Design review of the part built by this model. Coordinates are the model's own, in mm. A direction names the side the tool comes from. Give positions to 0.01 mm unless a question says otherwise; leave off trailing zeros. Order: outer loops, then holes, each group sorted by start corner. A loop starts at its lowest first (then second) coordinate and runs counter-clockwise, first axis right, second up. Notation, with made-up numbers: (64.25, 42.5) -> (77.25, 42.5) arc R16 ccw to (77.25, 51.5) -> close; hole circle Ø10 at (25, 60.25). An arc over 180 degrees is marked (long way). One line per item, written item: value. Start each with the question number.
1) The part is to be moulded in two halves that separate along Y. For faces 1 (the face through (2.958, 6.293, -6.36)), 2 (the face through (2.958, 3.735, 8.095)), 3 (the face through (2.958, -8.064, -3.8)), say which applies: released by +Y, released by -Y, zero draft, split by the parting line, or undercut.
2) Wall thickness on line 1 along Y through (x, z) = (2.1, 0); line 2 along Y through (x, z) = (0.35, 9.25); line 3 along Z through (x, y) = (2.05, 8.25): over which ranges is each line inside the solid? List them lowest first. Write a range as from..to.
3) Consider section D-D (y = 4). State the section outline as (x, z) points, plus the area to 3 significant figures.
4) Tool access review of faces 4 (the face through (2.96, -7.75, 0.01)), 5 (the face through (2.958, -3.881, -6.707)), 6 (the face through (2.958, 8.878, 0.813)), 7 (the face through (2.96, -2.34, 8.6)), 8 (the face through (6, 2.1, 2.4)): name each direction out of +Z, -Z, +X, -X, +Y, -Y from which nothing blocks a thin tool from reaching the whole face with its end or side.
5) Consider section B-B (y = 0). State the section outline as (x, z) points.
6) Consider section C-C (z = -3.75). State the section outline as (x, y) points.
7) Consider section A-A (z = 0). State the section outline as (x, y) points, plus the area to 3 significant figures.
from build123d import *

# Parameters (mm, degrees)
BASPROSKE_W        = 6
BASPROSKE_H        = 10
TOOTHCUT_DEPTH     = 16.362291496
TEETHCUTS_COUNT    = 18
TEETHCUTS_ANGLE    = 340
CUT_EXTRUDE1_DEPTH = 16.289512146


with BuildPart() as part:
    # BasProSke → Base-Revolve (revolve)
    with BuildSketch(Plane(origin=(0, 0, 0), x_dir=(1, 0, 0), z_dir=(0, 1, 0)), mode=Mode.PRIVATE) as base_revolve_sk:
        with Locations((3, 5)):
            Rectangle(BASPROSKE_W, BASPROSKE_H)
    revolve(base_revolve_sk.sketch.rotate(Axis((-10, 0, 0), (1, 0, 0)), 180), axis=Axis((-10, 0, 0), (1, 0, 0)))

    # TooCutSke → ToothCut (cut, through all)
    with BuildSketch(Plane(origin=(0, 0, 0), x_dir=(0, 0, -1), z_dir=(1, 0, 0))):
        with BuildLine():
            ThreePointArc((0.510641536, 7.732156635), (0, 7.749), (-0.510641536, 7.732156635))
            ThreePointArc((-0.510641536, 7.732156635), (-0.82619259, 8.907320741), (-1.515208602, 9.910236529))
            ThreePointArc((-1.515208602, 9.910236529), (0, 10.0254), (1.515208602, 9.910236529))
            ThreePointArc((1.515208602, 9.910236529), (0.82619259, 8.907320741), (0.510641536, 7.732156635))
        make_face()
    toothcut = extrude(amount=TOOTHCUT_DEPTH, mode=Mode.SUBTRACT)

    # TeethCuts: ToothCut ×18 about axis
    teethcuts_axis = Axis((-10, 0, 0), (1, 0, 0))
    for i in range(1, TEETHCUTS_COUNT):
        add(toothcut.rotate(teethcuts_axis, i * TEETHCUTS_ANGLE / (TEETHCUTS_COUNT - 1)), mode=Mode.SUBTRACT)

    # Sketch1 → Cut-Extrude1 (cut, through all)
    with BuildSketch(Plane(origin=(6, 0, 0), x_dir=(0, 0, -1), z_dir=(1, 0, 0))):
        with BuildLine():
            Line((2.374868417, 1.75), (2.374868417, -1.75))
            ThreePointArc((2.374868417, -1.75), (-2.95, 0), (2.374868417, 1.75))
        make_face()
    extrude(amount=-CUT_EXTRUDE1_DEPTH, mode=Mode.SUBTRACT)


solid = part.part
Checked values:
1. face 1: released by +Y
1. face 2: undercut
1. face 3: released by -Y
2. line 1: y = -7.75..-2.95, 2.95..7.75
2. line 2: y = -3.66..-2.91, -0.63..0.63, 2.91..3.66
2. line 3: z = -5.22..-3.99, -2.28..-0.6, 0.6..2.28, 3.99..5.22
3. outline: (0, -6.64) -> (6, -6.64) -> (6, 6.64) -> (0, 6.64) -> close
3. area: 79.6 mm^2
4. face 4: +X, -X, -Y
4. face 5: +X, -X
4. face 6: +X, -X, +Y
4. face 7: +Z, +X, -X
4. face 8: +Z, -Z, +X, +Y, -Y
5. outline: (0, -10) -> (6, -10) -> (6, -2.37) -> (0, -2.37) -> close; (0, 2.95) -> (6, 2.95) -> (6, 10) -> (0, 10) -> close
6. outline: (0, -8.01) -> (6, -8.01) -> (6, 8.01) -> (0, 8.01) -> close
7. outline: (0, -7.75) -> (6, -7.75) -> (6, -2.95) -> (0, -2.95) -> close; (0, 2.95) -> (6, 2.95) -> (6, 7.75) -> (0, 7.75) -> close
7. area: 57.6 mm^2
